Autodesk Inventor part; units mm, degrees
ref_plane "YZ Plane" through (0, 0, 0) normal (1, 0, 0) x (0, 1, 0)
ref_plane "XZ Plane" through (0, 0, 0) normal (0, 1, 0) x (-1, 0, 0)
ref_plane "XY Plane" through (0, 0, 0) normal (0, 0, 1) x (1, 0, 0)
sketch "Sketch1" plane through (0, 0, 0) normal (0, 0, 1) x (1, 0, 0)
  circle A0 centre (0, 0) radius 1.905
  circle A1 centre (0, 0) radius 3.3655
  line L0 (0, 0) -> (0, 28.575)
  line L1 (0, 0) -> (28.575, 0) construction
  circle A2 centre (0, 28.575) radius 32.639
  line L2 (0, 0) -> (6.35, 0)
  line L3 (6.35, 0) -> (-6.35, 0)
  circle A3 centre (-6.35, 0) radius 1.5875
  circle A4 centre (6.35, 0) radius 1.5875
  line L4 (0, 28.575) -> (11.1632, -2.0956)
  line L5 (0, 28.575) -> (32.639, 28.575) construction
  line L6 (0, 28.575) -> (-11.1632, -2.0956)
  circle A5 centre (0, 28.575) radius 23.8125
  dimension "d0" = 3.81
  dimension "d1" = 6.731
  dimension "d3" = 28.575
  dimension "d4" = 90
  dimension "d5" = 65.278
  dimension "d6" = 6.35
  dimension "d7" = 12.7
  dimension "d8" = 3.175
  dimension "d9" = 3.175
  dimension "d10" = 70
  dimension "d11" = 47.625
extrude "Extrusion1" add sketch "Sketch1" against normal blind 3.175 contours L2 A1 L3 A0 | A0 L0 A1 L2 | A0 L3 A1 L0 | A5 L4 A2 L6 | A5 L6 L0 | L0 L4 A5 picked at (-9.0211, 1.6136)
extrude "Extrusion2" cut sketch "Sketch1" against normal blind 1.905 contours L2 A1 L3 A0 | A0 L0 A1 L2 | A0 L3 A1 L0
extrude "Extrusion3" cut sketch "Sketch1" against normal through all contours A5 L6 L0 | L0 L4 A5 | L6 A5 L4
chamfer "Chamfer1" distance 1.27 angle 45 2 edges at (4.7625, 0, -3.175) (-7.9375, 0, -3.175)
fillet "Fillet1" radius 1.5875 4 edges at (8.1444, 6.1986, -1.5875) (11.1632, -2.0956, -1.5875) (-8.1444, 6.1986, -1.5875) (-11.1632, -2.0956, -1.5875)
equation "\"d9\" = d8"
properties part number "pushSwitchBushingHolder" material "ABS Plastic"
For this review, take the finished solid that the model builds, in its own axes (mm). A direction names the side the tool comes from. Give positions to 0.01 mm unless a question says otherwise; leave off trailing zeros. Order: outer loops, then holes, each group sorted by start corner. A loop starts at its lowest first (then second) coordinate and runs counter-clockwise, first axis right, second up.
1) Take a section at C-C (y = 5). Give the boundary of the cut face in (x, z) (3 decimals), then the cut area to 3 significant figures.
2) Insertion check: pin 1 (3.5 mm diameter, centred on x = 0, y = -1, fed in from +Z) (3 decimals); pin 2 (2.5 mm diameter, centred on x = 0, y = 0, fed in from +Z); pin 3 (4 mm diameter, centred on x = -6.35, y = 0, fed in from -Z). Each pin has a flat end and moves straight along its axis. Give the tip position at first contact, or say it passes through.
3) Take a section at B-B (x = -6.35). Give the boundary of the cut face in (y, z) (1 decimal), then the cut area to 3 significant figures.
4) Take a section at A-A (z = -0.6). State how many separate pieces and enclosed holes the cut face has, then the cut area to 3 significant figures.
5) The part is to be moulded in two halves that separate along X. For faces 4 (the face through (2, 1, -3.175)), 5 (the face through (0, -2.2, -1.905)), 6 (the face through (-0.136, -4.064, -1.565)), say which applies: released by +X, released by -X, zero draft, split by the parting line, or undercut.
6) For faces 1 (the face through (6.39, -1.81, -2.13)), 2 (the face through (2, 3, 0)), 3 (the face through (-2.67, -2.05, -0.94)), list the 3-axis set-ups (+Z, -Z, +X, -X, +Y, -Y) from which the entire face can be reached by the end or side of a thin tool; tool diameter is ignored.
7) Wall thickness on line 1 (Y direction, x = 0, z = -2.4) (1 decimal); line 2 (X direction, y = 0, z = -2.4) (1 decimal); line 3 (Z direction, x = 3, y = -0.5) (3 decimals): over which ranges is each line inside the solid? List them lowest first.
8) Take a section at D-D (x = 3). Give the boundary of the cut face in (y, z) (3 decimals), then the cut area to 3 significant figures.
Derived:
1. outline: (-8.556, -3.175) - (-3.355, -3.175) - (-3.355, 0) - (-8.556, 0) - close; (3.355, -3.175) - (8.556, -3.175) - (8.556, 0) - (3.355, 0) - close
1. area: 33.0 mm2
2. pin 1: stops at z = -1.905
2. pin 2: passes through
2. pin 3: stops at z = -2.32
3. outline: (-3.4, -3.2) - (-2.9, -3.2) - (-1.6, -1.9) - (-1.6, 0) - (-3.4, 0) - close; (1.6, -1.9) - (2.9, -3.2) - (5.6, -3.2) - (5.6, 0) - (1.6, 0) - close
3. area: 17.1 mm2
4. separate pieces: 1
4. enclosed holes: 3
4. area: 120 mm2
5. face 4: zero draft
5. face 5: undercut
5. face 6: split by the parting line
6. face 1: -Z
6. face 2: +Z, +X, -X, +Y, -Y
6. face 3: +Z
7. line 1: y = -4.1 to -1.9, 1.9 to 4.8
7. line 2: x = -10.4 to -8.4, -4.3 to -1.9, 1.9 to 4.3, 8.4 to 10.4
7. line 3: z = -3.175 to -1.905
8. outline: (-3.926, -3.175) - (4.952, -3.175) - (4.952, 0) - (1.525, 0) - (1.525, -1.905) - (-1.525, -1.905) - (-1.525, 0) - (-3.926, 0) - close
8. area: 22.4 mm2
